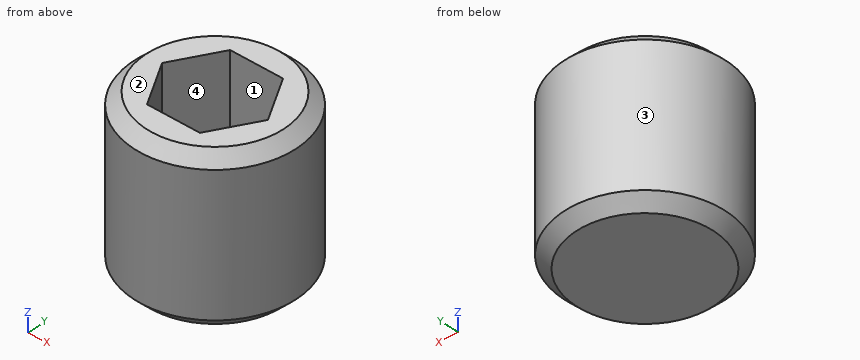
Solid Edge part; units mm, degrees
sketch "Sketch1" plane through (0, 0, 0) normal (0, 0, 1) x (1, 0, 0)
  circle A0 centre (0, 0) radius 12.7
extrude "Protrusion1" add sketch "Sketch1" along normal blind 25.4
chamfer "Chamfer1" distance 1.905 angle 45 2 edges at (-12.7, 0, 0) (-12.7, 0, 25.4)
sketch "Sketch2" plane through (0, 0, 25.4) normal (0, 0, 1) x (1, 0, 0)
  line L0 (-4.1244, 7.1438) -> (4.1244, 7.1438)
  line L1 (8.2489, 0) -> (4.1244, 7.1437)
  line L2 (4.1244, -7.1437) -> (8.2489, 0)
  line L3 (-4.1244, -7.1438) -> (4.1244, -7.1438)
  line L4 (-8.2489, 0) -> (-4.1244, -7.1437)
  line L5 (-4.1244, 7.1437) -> (-8.2489, 0)
extrude "Cutout1" cut sketch "Sketch2" against normal blind 12.7
properties part number "24103863"
Check sheet for the modelled part. Datum: model origin and axes. Units: mm. Face numbers are marked on the shaded views. Round coordinates to 2 decimals unless told otherwise and drop trailing zeros. Loops run counter-clockwise (first coordinate to the right, second up) from the corner with the lowest first, then second, coordinate; pieces in that order, holes last. Notation, with made-up numbers: (69.5, 34.5) -> (113.5, 34.5) arc R33 cw to (113.5, 63.5) -> close; hole circle Ø6 at (56, 47). An arc over 180 degrees is marked (long way). Put each result on its own line as item: value. Start each with the question number.
1. Section check A-A (z = 13.25). Enter the section's corners in (x, y), plus the area to 3 significant figures.
2. Gauge pin test, flat ends, axial feed: pin 1 (4 mm diameter, centred on y = -2, z = 13, fed in from +X); pin 2 (2 mm diameter, centred on x = 0.5, y = -4.5, fed in from +Z); pin 3 (5 mm diameter, centred on y = -4, z = 18, fed in from +X); pin 4 (6 mm diameter, centred on x = 9.5, z = 9, fed in from +Y). Record the tip position at first contact, or that the pin passes through.
3. Scan lines: probe 1 along Y at (x, z) = (3.75, 17.5); probe 2 along Y at (x, z) = (2.75, 16); probe 3 along Z at (x, y) = (-6, -2.75). Record each from-to range of solid material in increasing order.
4. Section check C-C (z = 6.5). Enter the section's corners in (x, y), plus the area to 3 significant figures.
5. Section check B-B (x = 0). Enter the section's corners in (y, z) (3 decimals).
6. Draft check along X on the marked faces 1, 2, 3 and 4. Enter one of: +X half, -X half, draft (parallel to the pull), parting line (faces both ways), or undercut.
Findings:
1. outline: circle Ø25.4 at (0, 0); hole (-8.25, 0) -> (-4.12, -7.14) -> (4.12, -7.14) -> (8.25, 0) -> (4.12, 7.14) -> (-4.12, 7.14) -> close
1. area: 330 mm^2
2. pin 1: stops at x = 12.7
2. pin 2: stops at z = 12.7
2. pin 3: stops at x = 12.61
2. pin 4: stops at y = 10.91
3. probe 1: y = -12.13 to -7.14, 7.14 to 12.13
3. probe 2: y = -12.4 to -7.14, 7.14 to 12.4
3. probe 3: z = 0 to 12.7
4. outline: circle Ø25.4 at (0, 0)
4. area: 507 mm^2
5. outline: (-12.7, 1.905) -> (-10.795, 0) -> (10.795, 0) -> (12.7, 1.905) -> (12.7, 23.495) -> (10.795, 25.4) -> (7.144, 25.4) -> (7.144, 12.7) -> (-7.144, 12.7) -> (-7.144, 25.4) -> (-10.795, 25.4) -> (-12.7, 23.495) -> close
6. face 1: undercut
6. face 2: draft
6. face 3: parting line
6. face 4: undercut
